Autodesk Inventor part; units mm, degrees
ref_plane "YZ Plane" through (0, 0, 0) normal (1, 0, 0) x (0, 1, 0)
ref_plane "XZ Plane" through (0, 0, 0) normal (0, 1, 0) x (-1, 0, 0)
ref_plane "XY Plane" through (0, 0, 0) normal (0, 0, 1) x (1, 0, 0)
sketch "Sketch1" plane through (0, 0, 0) normal (0, 1, 0) x (-1, 0, 0)
  line L0 (51.5704, 31.4309) -> (74.021, 53.8815)
  line L1 (74.021, 53.8815) -> (109.942, 17.9605)
  line L2 (109.942, 17.9605) -> (100.9618, 8.9803)
  line L3 (100.9618, 8.9803) -> (74.021, 35.921)
  line L4 (74.021, 35.921) -> (47.0803, 8.9803)
  line L5 (100.9618, 8.9803) -> (107.5624, 2.3796) construction
  line L6 (35.9043, 29.2241) -> (44.6165, 29.2241) construction
  line L7 (35.9043, 29.2241) -> (27.1921, 29.2241) construction
  circle A0 centre (44.6165, 29.2241) radius 1.5263
  circle A1 centre (27.1921, 29.2241) radius 1.6891
  circle A2 centre (35.9043, 20.4103) radius 2.54
  circle A3 centre (35.9043, 8.9803) radius 6.35
  line L8 (51.5704, 31.4309) -> (51.5704, 36.1902)
  line L9 (51.5704, 36.1902) -> (22.0986, 36.1902)
  line L10 (22.0986, 36.1902) -> (22.0986, 17.9605)
  line L11 (47.0803, 8.9803) -> (47.0803, 0)
  line L12 (5.5886, 17.9605) -> (22.0986, 17.9605)
  line L13 (5.5886, 17.9605) -> (5.5886, -7.4395)
  line L14 (5.5886, -7.4395) -> (47.0803, -7.4395)
  line L15 (47.0803, -7.4395) -> (47.0803, 0)
  point P0 (0, 0)
  dimension "d1" = 12.7
  dimension "d3" = 38.1
  dimension "d5" = 12.7
  dimension "d19" = 8.7122
  dimension "d20" = 8.7122
  dimension "d23" = 5.08
  dimension "d24" = 25.4
  dimension "d38" = 16.51
  dimension "d39" = 29.4718
extrude "Extrusion1" add sketch "Sketch1" along normal blind 5.08
sketch "Sketch2" plane through (0, 5.08, 0) normal (0, 1, 0) x (1, 0, 0)
  line L0 (-5.5886, -17.9605) -> (-5.5886, 7.4395)
  line L1 (-13.1234, -2.7205) -> (-13.1234, -7.8005)
  line L2 (-13.1234, -5.2605) -> (-2.9634, -5.2605) construction
  line L3 (-5.5886, 7.4395) -> (-47.0803, 7.4395) construction
  line L4 (-22.0986, -17.9605) -> (-5.5886, -17.9605) construction
  line L5 (-13.1234, -7.8005) -> (-2.9634, -7.8005)
  line L6 (-2.9634, -7.8005) -> (-2.9634, -2.7205)
  line L7 (-2.9634, -2.7205) -> (-13.1234, -2.7205)
  line L8 (-13.1234, -2.7205) -> (-13.1234, -7.8005)
  line L9 (-47.0803, 7.4395) -> (-47.0803, -8.9803)
  point P0 (0, 0)
  point P1 (-5.5886, -2.7205)
  point P2 (-5.5886, -7.8005)
  dimension "d29" = 5.08
  dimension "d30" = 12.7
  dimension "d31" = 25.4
  dimension "d40" = 33.9568
  dimension "d41" = 10.16
extrude "Extrusion2" cut sketch "Sketch2" against normal blind 25.4 contours L5 L1 L7 L0
sketch "Sketch3" plane through (0, 5.08, 0) normal (0, 1, 0) x (1, 0, 0)
  circle A0 centre (-19.4734, -5.2605) radius 1.4605
  line L0 (-13.1234, -7.8005) -> (-13.1234, -2.7205)
  line L1 (-13.1234, -5.2605) -> (-2.0744, -5.2605) construction
  point P0 (0, 0)
  dimension "d34" = 6.35
  dimension "d35" = 2.921
extrude "Extrusion3" cut sketch "Sketch3" against normal blind 25.4
sketch "Sketch4" plane through (0, 5.08, 0) normal (0, 1, 0) x (1, 0, 0)
  circle A0 centre (-19.4734, -5.2605) radius 1.4605
  line L0 (-13.1234, -2.7205) -> (-5.5886, -2.7205)
  line L1 (-5.5886, -2.7205) -> (-5.5886, 7.4395)
  line L2 (-5.5886, 7.4395) -> (-47.0803, 7.4395)
  line L3 (-47.0803, 7.4395) -> (-47.0803, -8.9803)
  line L4 (-47.0803, -8.9803) -> (-74.021, -35.921)
  line L5 (-74.021, -35.921) -> (-100.9618, -8.9803)
  line L6 (-100.9618, -8.9803) -> (-109.942, -17.9605)
  line L7 (-109.942, -17.9605) -> (-74.021, -53.8815)
  line L8 (-74.021, -53.8815) -> (-51.5704, -31.4309)
  line L9 (-51.5704, -31.4309) -> (-51.5704, -36.1902)
  line L10 (-51.5704, -36.1902) -> (-22.0986, -36.1902)
  line L11 (-22.0986, -36.1902) -> (-22.0986, -17.9605)
  line L12 (-22.0986, -17.9605) -> (-5.5886, -17.9605)
  line L13 (-5.5886, -17.9605) -> (-5.5886, -7.8005)
  line L14 (-5.5886, -7.8005) -> (-13.1234, -7.8005)
  line L15 (-13.1234, -7.8005) -> (-13.1234, -2.7205)
  circle A1 centre (-44.6165, -29.2241) radius 1.5263
  circle A2 centre (-27.1921, -29.2241) radius 1.6891
  circle A3 centre (-35.9043, -20.4103) radius 2.54
  circle A4 centre (-35.9043, -8.9803) radius 6.35
  point P0 (0, 0)
properties part number "gripper laser cut"
Work out the finished part from the listing and answer in its coordinate system (mm). A direction names the side the tool comes from. Give positions to 0.01 mm unless a question says otherwise; leave off trailing zeros. Write each loop counter-clockwise with the first axis right and the second up, starting at its lowest first coordinate (ties: lowest second). Pieces come first, ordered by that corner, then holes.
Q1. The part is cut by section D-D on z = 1. Give the vertices of the cut face in (x, y), and give its area (3 significant figures).
Answer:
outline: (-47.08, 0) - (-5.59, 0) - (-5.59, 5.08) - (-47.08, 5.08) - close
area: 211 mm2
Q2. The part is cut by section A-A on z = 33. Give the vertices of the cut face in (x, y), and give its area (3 significant figures).
Answer:
outline: (-94.9, 0) - (-76.94, 0) - (-76.94, 5.08) - (-94.9, 5.08) - close; (-71.1, 0) - (-53.14, 0) - (-53.14, 5.08) - (-71.1, 5.08) - close; (-51.57, 0) - (-22.1, 0) - (-22.1, 5.08) - (-51.57, 5.08) - close
area: 332 mm2
Q3. The part is cut by section B-B on x = -50.5. Give the vertices of the cut face in (y, z), and give its area (3 significant figures).
Answer:
outline: (0, 12.4) - (5.08, 12.4) - (5.08, 36.19) - (0, 36.19) - close
area: 121 mm2
Q4. Straight lines are drawn through the part: L1, parallel to Z at x = -13, y = 1.1; L2, parallel to Z at x = -37, y = 4.85; L3, parallel to X at y = 4.45, z = 14.5. For each, find the intervals that lie inside material, in ascending order.
Answer:
L1: z = -7.44 to 2.72, 7.8 to 17.96
L2: z = -7.44 to 2.73, 15.24 to 18.12, 22.7 to 36.19
L3: x = -106.48 to -95.44, -52.6 to -39.04, -32.76 to -5.59
Q5. For a pull along X with two mould halves and no side action, classify faces 1 (the face through (-5.589, 3, -2)), 2 (the face through (-14, 3, 17.96)), 3 (the face through (-51.57, 3, 34)) as released by +X, released by -X, zero draft, split by the parting line, or undercut.
Answer:
face 1: released by +X
face 2: zero draft
face 3: undercut
Q6. Given pin 1 (1.5 mm diameter, centred on y = 3.5, z = 26, fed in from +X); pin 2 (1 mm diameter, centred on x = -96.5, z = 27.5, fed in from -Y); pin 3 (2.5 mm diameter, centred on y = 3, z = 5, fed in from +X); pin 4 (1.5 mm diameter, centred on x = -97, y = 2.5, fed in from -Z), each flat-ended and moving along its own axis, determine where each tip first touches the part or whether it passes through.
Answer:
pin 1: stops at x = -22.1
pin 2: stops at y = 0
pin 3: stops at x = -13.12
pin 4: stops at z = 12.19
Q7. A tool of negligible diameter and unlimited length cuts with its end or side. For faces 4 (the face through (-87.68, 2.5, 22.26)), 5 (the face through (-37, 3, 36.19)), 6 (the face through (-62.64, 2.5, 42.5)), 7 (the face through (-47.08, 3, 1)), 8 (the face through (-9, 3, 2.72)), from which of +Z, -Z, +X, -X, +Y, -Y can it reach the whole face along a straight path? Write none if from no direction.
Answer:
face 4: -Z, +Y, -Y
face 5: +Z, +X, +Y, -Y
face 6: +Z, +Y, -Y
face 7: -Z, -X, +Y, -Y
face 8: +X, +Y, -Y
Q8. The part is cut by section C-C on y = 1.3. Give the vertices of the cut face in (x, z), and give its area (3 significant figures).
Answer:
outline: (-109.94, 17.96) - (-100.96, 8.98) - (-74.02, 35.92) - (-47.08, 8.98) - (-47.08, -7.44) - (-5.59, -7.44) - (-5.59, 2.72) - (-13.12, 2.72) - (-13.12, 7.8) - (-5.59, 7.8) - (-5.59, 17.96) - (-22.1, 17.96) - (-22.1, 36.19) - (-51.57, 36.19) - (-51.57, 31.43) - (-74.02, 53.88) - close; hole circle Ø3.05 at (-44.62, 29.22); hole circle Ø12.7 at (-35.9, 8.98); hole circle Ø5.08 at (-35.9, 20.41); hole circle Ø3.38 at (-27.19, 29.22); hole circle Ø2.92 at (-19.47, 5.26)
area: 2,380 mm2
